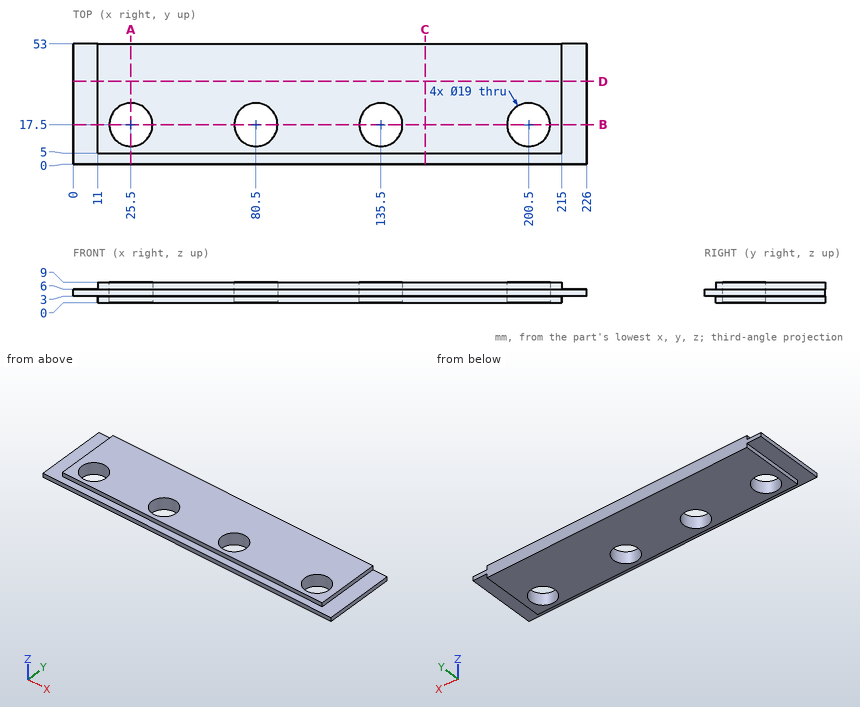
Geometry check sheet. Reference: drawing and pictorial views, mm from the part's lowest x, y, z. Give positions to 0.01 mm unless a question says otherwise; leave off trailing zeros. Order: outer loops, then holes, each group sorted by start corner. A loop starts at its lowest first (then second) coordinate and runs counter-clockwise, first axis right, second up. Notation, with made-up numbers: M 61.5,19.5 L 96.5,19.5 A15 ccw 96.5,31.5 Z; hole C 88.5,38.5 d4. An arc over 180 degrees is marked long. Use one line per item in the form item = value. Start each with the question number.
Q1. Scan lines: line 1 along X through (y, z) = (17, 5.5); line 2 along X through (y, z) = (24.5, 8); line 3 along Y through (x, z) = (200.5, 6.25). Record each from-to range of solid material in increasing order. Write a range as [from, to].
Q2. Section check B-B (y = 17.5). Enter the section's corners in (x, z).
Q3. Section check C-C (x = 155). Enter the section's corners in (y, z), then the cut area to 3 significant figures.
Q4. Go/stop test with flat-tipped pins: pin 1 Ø0.9 at (x, z) = (153.5, 1.5) entering from -Y; pin 2 Ø0.9 at (y, z) = (20.5, 7) entering from +X; pin 3 Ø3.5 at (y, z) = (24, 1) entering from -X; pin 4 Ø15 at (x, y) = (25.5, 17.5) entering from -Z. Record where each tip stops, or that it passes through.
Q5. Section check D-D (y = 36.5). Enter the section's corners in (x, z).
Q6. Section check A-A (x = 25.5). Enter the section's corners in (y, z), then the cut area to 3 significant figures.
Evaluation:
q1.line_1 = [0, 16.01], [34.99, 71.01], [89.99, 126.01], [144.99, 191.01], [209.99, 226]
q1.line_2 = [11, 19.08], [31.92, 74.08], [86.92, 129.08], [141.92, 194.08], [206.92, 215]
q1.line_3 = [5, 8], [27, 53]
q2.outline = M 0,3 L 11,3 L 11,0 L 16,0 L 16,9 L 11,9 L 11,6 L 0,6 Z; M 35,0 L 71,0 L 71,9 L 35,9 Z; M 90,0 L 126,0 L 126,9 L 90,9 Z; M 145,0 L 191,0 L 191,9 L 145,9 Z; M 210,0 L 215,0 L 215,3 L 226,3 L 226,6 L 215,6 L 215,9 L 210,9 Z
q3.outline = M 0,3 L 5,3 L 5,0 L 53,0 L 53,9 L 5,9 L 5,6 L 0,6 Z
q3.area = 447 mm2
q4.pin_1 = 5
q4.pin_2 = 215
q4.pin_3 = 11
q4.pin_4 = through
q5.outline = M 0,3 L 11,3 L 11,0 L 215,0 L 215,3 L 226,3 L 226,6 L 215,6 L 215,9 L 11,9 L 11,6 L 0,6 Z
q6.outline = M 0,3 L 5,3 L 5,0 L 8,0 L 8,9 L 5,9 L 5,6 L 0,6 Z; M 27,0 L 53,0 L 53,9 L 27,9 Z
q6.area = 276 mm2
